Could you check a few things on this model? Use its own coordinates, in mm. Face numbers are marked on the shaded views. A direction names the side the tool comes from. Give positions to 0.01 mm unless a question says otherwise; leave off trailing zeros. Write each loop counter-clockwise with the first axis right and the second up, starting at its lowest first coordinate (ties: lowest second). Pieces come first, ordered by that corner, then holes. Notation, with made-up numbers: (81, 70.5) - (136, 70.5) arc R29 ccw to (136, 99.5) - close; hole circle Ø9 at (44.25, -38). An arc over 180 degrees is marked (long way). Answer in a Markdown table with one row per item.
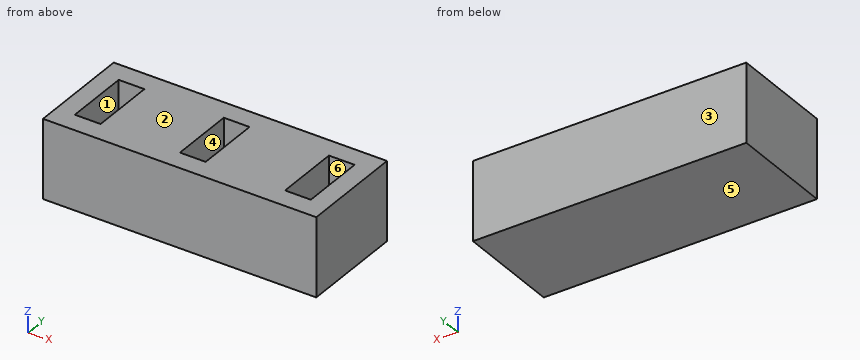
from build123d import *

# Parameters (mm, degrees)
BOX003_W     = 4.9
BOX003_H     = 12.4
BOX003_DEPTH = 10
BOX002_W     = 4.9
BOX002_H     = 12.4
BOX002_DEPTH = 10
BOX001_W     = 4.9
BOX001_H     = 12.4
BOX001_DEPTH = 10
BOX_W        = 52
BOX_H        = 20
BOX_DEPTH    = 15


with BuildPart() as cubo003:
    # Box003 → Box003 (new body)
    with BuildSketch(Plane(origin=(43.5, 3.8, 5), x_dir=(1, 0, 0), z_dir=(0, 0, 1))):
        with Locations((2.45, 6.2)):
            Rectangle(BOX003_W, BOX003_H)
    extrude(amount=BOX003_DEPTH)


with BuildPart() as cubo002:
    # Box002 → Box002 (new body)
    with BuildSketch(Plane(origin=(23.5, 3.8, 5), x_dir=(1, 0, 0), z_dir=(0, 0, 1))):
        with Locations((2.45, 6.2)):
            Rectangle(BOX002_W, BOX002_H)
    extrude(amount=BOX002_DEPTH)


with BuildPart() as cubo001:
    # Box001 → Box001 (new body)
    with BuildSketch(Plane(origin=(3.5, 3.8, 5), x_dir=(1, 0, 0), z_dir=(0, 0, 1))):
        with Locations((2.45, 6.2)):
            Rectangle(BOX001_W, BOX001_H)
    extrude(amount=BOX001_DEPTH)


with BuildPart() as cut002:
    # Box → Box (new body)
    with BuildSketch(Plane.XY):
        with Locations((26, 10)):
            Rectangle(BOX_W, BOX_H)
    extrude(amount=BOX_DEPTH)

    # Cut: cut Cubo001
    add(cubo001.part, mode=Mode.SUBTRACT)

    # Cut001: cut Cubo002
    add(cubo002.part, mode=Mode.SUBTRACT)

    # Cut002: cut Cubo003
    add(cubo003.part, mode=Mode.SUBTRACT)


solid = cut002.part
1) Imagine slicing it at A-A (z = 11.25). List the corners of the cut face in (x, y) for me, then the cut area to 3 significant figures.
Check values:
| item | result |
|---|---|
| outline | (0, 0) - (52, 0) - (52, 20) - (0, 20) - close; hole (3.5, 3.8) - (8.4, 3.8) - (8.4, 16.2) - (3.5, 16.2) - close; hole (23.5, 3.8) - (28.4, 3.8) - (28.4, 16.2) - (23.5, 16.2) - close; hole (43.5, 3.8) - (48.4, 3.8) - (48.4, 16.2) - (43.5, 16.2) - close |
| area | 858 mm2 |
2) We'd pull the mould along Y, two halves only. Please class the marked faces 3, 4, 5 and 6: +Y half, -Y half, draft (parallel to the pull), parting line (faces both ways), or undercut.
Check values:
| item | result |
|---|---|
| face 3 | +Y half |
| face 4 | undercut |
| face 5 | draft |
| face 6 | undercut |
3) If I drill on line 1 (X direction, y = 5, z = 13.25); line 2 (Z direction, x = 44, y = 16); line 3 (Y direction, x = 45, z = 9), over which ranges is the centre line in solid material (lowest first)?
Check values:
| item | result |
|---|---|
| line 1 | x = 0 to 3.5, 8.4 to 23.5, 28.4 to 43.5, 48.4 to 52 |
| line 2 | z = 0 to 5 |
| line 3 | y = 0 to 3.8, 16.2 to 20 |
4) Imagine slicing it at B-B (x = 25). List the corners of the cut face in (y, z) for me.
Check values:
| item | result |
|---|---|
| outline | (0, 0) - (20, 0) - (20, 15) - (16.2, 15) - (16.2, 5) - (3.8, 5) - (3.8, 15) - (0, 15) - close |
5) On a 3-axis mill with a long thin cutter (end or side, diameter ignored), from which of +Z, -Z, +X, -X, +Y, -Y can I reach the whole of each face in a straight line? I mean the marked faces 1 and 2. Say none if no direction works.
Check values:
| item | result |
|---|---|
| face 1 | +Z |
| face 2 | +Z, +X, -X, +Y, -Y |
6) Imagine slicing it at C-C (y = 14.5). List the corners of the cut face in (x, z) for me.
Check values:
| item | result |
|---|---|
| outline | (0, 0) - (52, 0) - (52, 15) - (48.4, 15) - (48.4, 5) - (43.5, 5) - (43.5, 15) - (28.4, 15) - (28.4, 5) - (23.5, 5) - (23.5, 15) - (8.4, 15) - (8.4, 5) - (3.5, 5) - (3.5, 15) - (0, 15) - close |
